Could you check a few things on this drawing? It's one solid part, dimensions in mm from its lowest x, y, z. A direction names the side the tool comes from. Give positions to 0.01 mm unless a question says otherwise; leave off trailing zeros. Order: outer loops, then holes, each group sorted by start corner. A loop starts at its lowest first (then second) coordinate and runs counter-clockwise, first axis right, second up. Notation, with made-up numbers: M 87.25,84 L 140.25,84 A9 ccw 140.25,95 Z; hole C 77,0.5 d1. An arc over 180 degrees is marked long. Use one line per item in the form item = value. Start each with the question number.
1. I want a section at B-B, the plane x = 102.5. List the corners of the cut face in (y, z) for me.
2. We'd pull the mould along Z, two halves only. Please class the marked faces 3, 4, 5 and 6: +Z half, -Z half, draft (parallel to the pull), parting line (faces both ways), or undercut.
3. For the marked faces 1 and 2, which set-ups out of +Z, -Z, +X, -X, +Y, -Y let a thin tool reach every point of the face, with its end or its side?
4. Will this pin go through, and if not, where does the flat tip stop? P1, Ø2, axis at x = 123, z = 155, coming from the +Y side.
5. I want a section at A-A, the plane y = 32.5. List the corners of the cut face in (x, z) for me, and give its area (3 significant figures).
6. I need wall thicknesses on L1, parallel to Z at x = 231.5, y = 71; L2, parallel to X at y = 30, z = 152; L3, parallel to Y at x = 283, z = 194. Which ranges of each line are inside material? Lowest first, please.
7. I want a section at C-C, the plane z = 31. List the corners of the cut face in (x, y) for me.
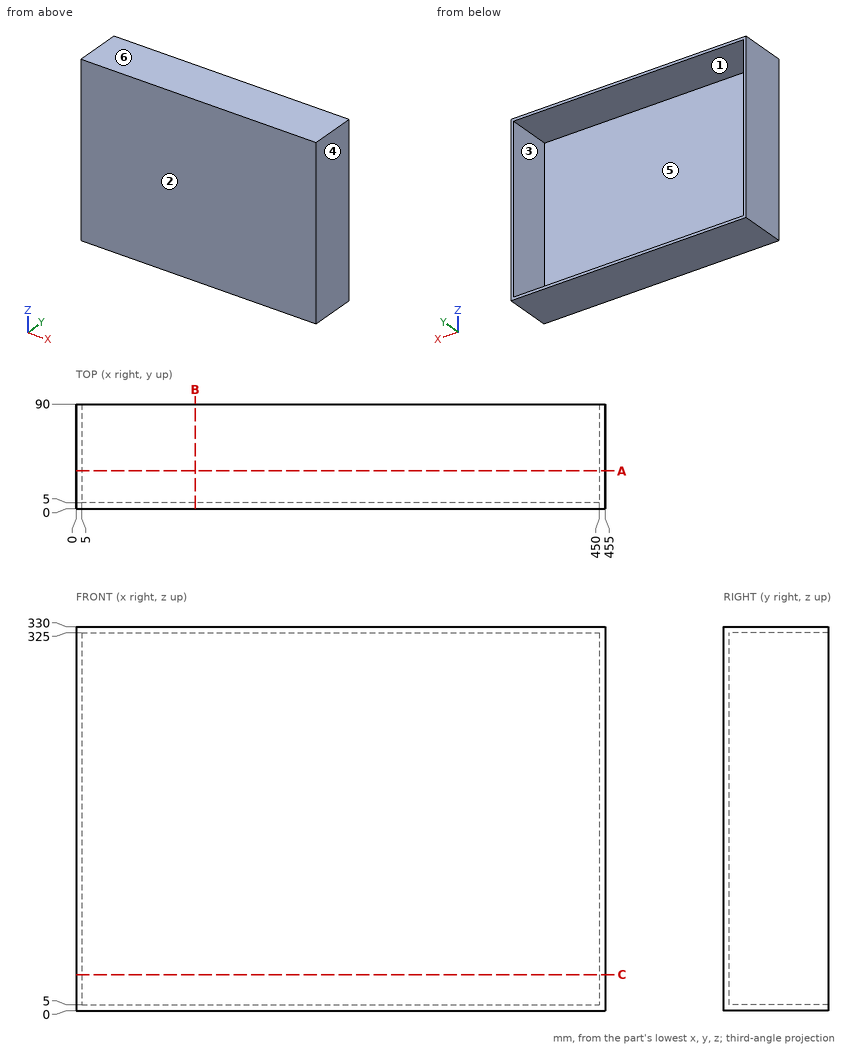
Check result:
q1.outline = M 0,0 L 90,0 L 90,5 L 5,5 L 5,325 L 90,325 L 90,330 L 0,330 Z
q2.face_3 = undercut
q2.face_4 = draft
q2.face_5 = undercut
q2.face_6 = +Z half
q3.face_1 = +Y
q3.face_2 = +Z, -Z, +X, -X, -Y
q4.P1 = 5
q5.outline = M 0,0 L 455,0 L 455,330 L 0,330 Z; hole M 5,5 L 450,5 L 450,325 L 5,325 Z
q5.area = 7,750 mm2
q6.L1 = 0 to 5, 325 to 330
q6.L2 = 0 to 5, 450 to 455
q6.L3 = 0 to 5
q7.outline = M 0,0 L 455,0 L 455,90 L 450,90 L 450,5 L 5,5 L 5,90 L 0,90 Z
